Check sheet for the drawn part. Datum: minimum x, y, z corner. Units: mm. A direction names the side the tool comes from. Round coordinates to 2 decimals unless told otherwise and drop trailing zeros. Order: outer loops, then holes, each group sorted by start corner. A loop starts at its lowest first (then second) coordinate and runs counter-clockwise, first axis right, second up. Notation, with made-up numbers: (58.5, 29) - (100.5, 29) arc R17 cw to (100.5, 51) - close; hole circle Ø10 at (82, -38.75). An arc over 180 degrees is marked (long way). Write each question's results on one line, items separated by ' | '.
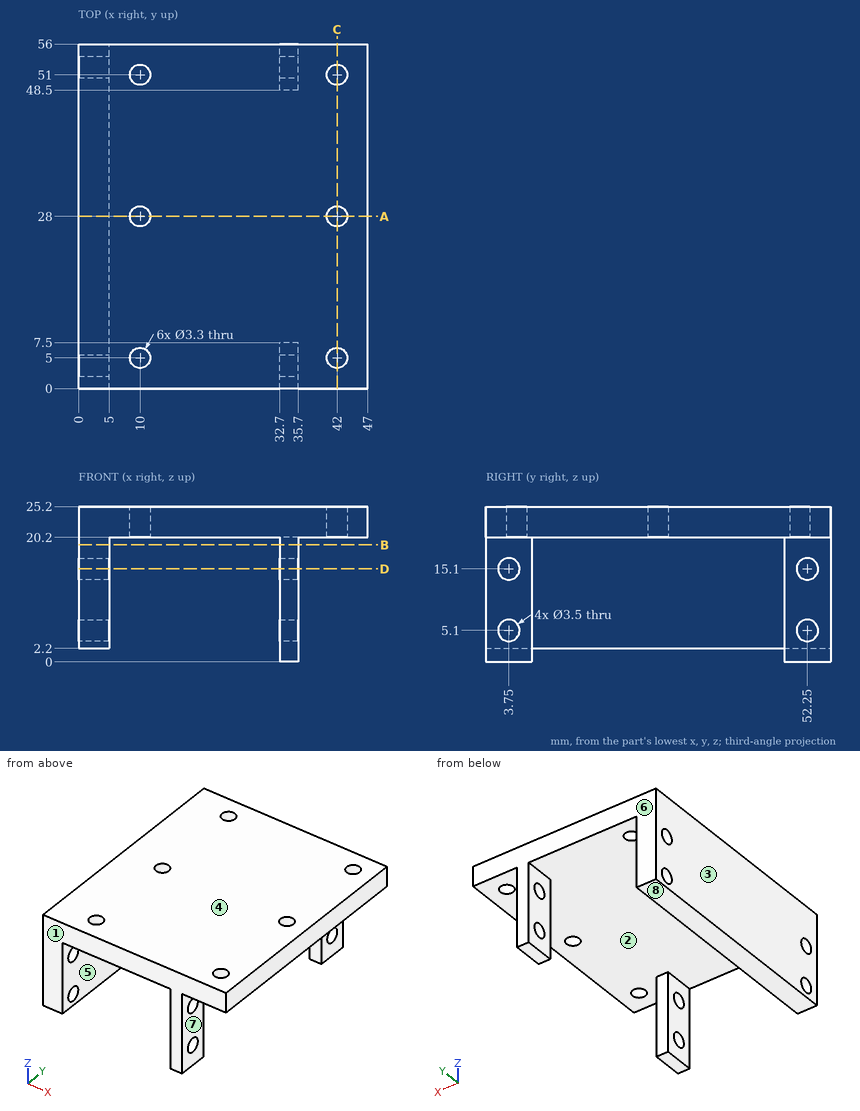
(1) Section check C-C (x = 42). Record the cut outline in (y, z).
Answers follow:
outline: (0, 20.2) - (3.35, 20.2) - (3.35, 25.2) - (0, 25.2) - close; (6.65, 20.2) - (26.35, 20.2) - (26.35, 25.2) - (6.65, 25.2) - close; (29.65, 20.2) - (49.35, 20.2) - (49.35, 25.2) - (29.65, 25.2) - close; (52.65, 20.2) - (56, 20.2) - (56, 25.2) - (52.65, 25.2) - close
(2) Draft check along X on the marked faces 1, 2 and 3. Enter one of: released by +X, released by -X, zero draft, split by the parting line, or undercut.
Answers follow:
face 1: zero draft | face 2: undercut | face 3: released by -X
(3) Section check A-A (y = 28). Record the cut outline in (x, z), then the cut area to 3 significant figures.
Answers follow:
outline: (0, 2.2) - (5, 2.2) - (5, 20.2) - (8.35, 20.2) - (8.35, 25.2) - (0, 25.2) - close; (11.65, 20.2) - (40.35, 20.2) - (40.35, 25.2) - (11.65, 25.2) - close; (43.65, 20.2) - (47, 20.2) - (47, 25.2) - (43.65, 25.2) - close | area: 292 mm²
(4) Section check B-B (z = 19). Record the cut outline in (x, y).
Answers follow:
outline: (0, 0) - (5, 0) - (5, 56) - (0, 56) - close; (32.7, 0) - (35.7, 0) - (35.7, 7.5) - (32.7, 7.5) - close; (32.7, 48.5) - (35.7, 48.5) - (35.7, 56) - (32.7, 56) - close
(5) Section check D-D (z = 15.1). Record the cut outline in (x, y), then the cut area to 3 significant figures.
Answers follow:
outline: (0, 0) - (5, 0) - (5, 2) - (0, 2) - close; (0, 5.5) - (5, 5.5) - (5, 50.5) - (0, 50.5) - close; (0, 54) - (5, 54) - (5, 56) - (0, 56) - close; (32.7, 0) - (35.7, 0) - (35.7, 2) - (32.7, 2) - close; (32.7, 5.5) - (35.7, 5.5) - (35.7, 7.5) - (32.7, 7.5) - close; (32.7, 48.5) - (35.7, 48.5) - (35.7, 50.5) - (32.7, 50.5) - close; (32.7, 54) - (35.7, 54) - (35.7, 56) - (32.7, 56) - close | area: 269 mm²
(6) Material ranges on line 1 (Y direction, x = 1.2, z = 5.1); line 2 (Y direction, x = 10, z = 22.1); line 3 (Z direction, x = 34, y = 52), recorded low to high.
Answers follow:
line 1: 0 to 2, 5.5 to 50.5, 54 to 56 | line 2: 0 to 3.35, 6.65 to 26.35, 29.65 to 49.35, 52.65 to 56 | line 3: 0 to 3.37, 6.83 to 13.37, 16.83 to 25.2
(7) Depth check by flat-ended pin: pin 1 Ø8 at (x, y) = (20.5, 21.5) entering from -Z; pin 2 Ø12 at (y, z) = (44.5, 10) entering from +X; pin 3 Ø1.5 at (x, y) = (1.5, 19.5) entering from -Z. Enter the tip coordinate at first touch or a pass-through.
Answers follow:
pin 1: z = 20.2 | pin 2: x = 35.7 | pin 3: z = 2.2
(8) Access from +Z, -Z, +X, -X, +Y, -Y to the whole of each face (thin tool, end or side, straight path). Record for the marked faces 4, 5, 6, 7 and 8.
Answers follow:
face 4: +Z, +X, -X, +Y, -Y | face 5: -Z, +Y, -Y | face 6: +Z, -Z, +X, -X, +Y | face 7: -Z, +X, +Y, -Y | face 8: -Z, -X, +Y, -Y
